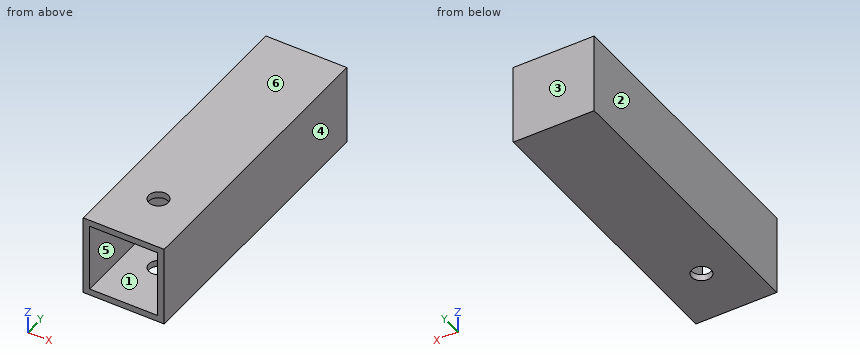
from build123d import *

# Parameters (mm, degrees)
SKETCH1_W                = 25.000000038
SKETCH1_H                = 25.000000038
BOSS_EXTRUDE1_DEPTH      = 120
SHELL1_T                 = -2
F_6_0_6_DIAMETER_HOLE1_D = 6
SKETCH6_W                = 35.234136461
SKETCH6_H                = 40.928418781
CUT_EXTRUDE1_DEPTH       = 48.26
SKETCH6_2_W              = 35.234136461
SKETCH6_2_H              = 40.928418781
CUT_EXTRUDE2_DEPTH       = 48.26
CUT_EXTRUDE2_DEPTH_BACK  = 48.26


with BuildPart() as part:
    # Sketch1 → Boss-Extrude1 (new body)
    with BuildSketch(Plane(origin=(0, 0, 0), x_dir=(1, 0, 0), z_dir=(0, 1, 0))):
        Rectangle(SKETCH1_W, SKETCH1_H)
    extrude(amount=BOSS_EXTRUDE1_DEPTH)

    # Shell1
    shell1_openings = [part.faces().sort_by_distance(p)[0] for p in [
        (0, 0, 0),
    ]]
    offset(amount=SHELL1_T, openings=shell1_openings, kind=Kind.INTERSECTION)

    # 6.0 _6_ Diameter Hole1 (through all)
    with Locations(Plane.XY.offset(12.500000019)):
        with Locations((0, 46.99999998)):
            Hole(F_6_0_6_DIAMETER_HOLE1_D / 2)

    # Sketch6 → Cut-Extrude1 (cut)
    with BuildSketch(Plane.XY):
        with Locations((1.431161847, 9.333336088)):
            Rectangle(SKETCH6_W, SKETCH6_H)
    extrude(amount=-CUT_EXTRUDE1_DEPTH, mode=Mode.SUBTRACT)

    # Sketch6_2 → Cut-Extrude2 (cut, two sides)
    with BuildSketch(Plane.XY) as cut_extrude2_sk:
        with Locations((1.431161847, 9.333336088)):
            Rectangle(SKETCH6_2_W, SKETCH6_2_H)
    extrude(amount=CUT_EXTRUDE2_DEPTH, mode=Mode.SUBTRACT)
    extrude(cut_extrude2_sk.sketch, amount=-CUT_EXTRUDE2_DEPTH_BACK, mode=Mode.SUBTRACT)


solid = part.part
Work out the finished part from the listing and answer in its coordinate system (mm). Face numbers are marked on the shaded views. A direction names the side the tool comes from. Round coordinates to 2 decimals unless told otherwise and drop trailing zeros. Write each loop counter-clockwise with the first axis right and the second up, starting at its lowest first coordinate (ties: lowest second). Pieces come first, ordered by that corner, then holes. Notation, with made-up numbers: M 85,49 L 126,49 A33 cw 126,85 Z; hole C -4.75,59 d5. An arc over 180 degrees is marked long. Use a Markdown table: item, result.
1) The part is cut by section A-A on x = 0. Give the vertices of the cut face in (y, z), plus the area to 3 significant figures.
Taken from the geometry:
| item | result |
|---|---|
| outline | M 29.8,-12.5 L 44,-12.5 L 44,-10.5 L 29.8,-10.5 Z; M 29.8,10.5 L 44,10.5 L 44,12.5 L 29.8,12.5 Z; M 50,-12.5 L 120,-12.5 L 120,12.5 L 50,12.5 L 50,10.5 L 118,10.5 L 118,-10.5 L 50,-10.5 Z |
| area | 379 mm2 |
2) Consider line 1 (Z direction, x = -10, y = 95.5); line 2 (Y direction, x = 0, z = -11.25); line 3 (X direction, y = 47, z = 11.45). Determine where each line is inside the solid, lowest interval first. Write a range as [from, to].
Taken from the geometry:
| item | result |
|---|---|
| line 1 | z = [-12.5, -10.5], [10.5, 12.5] |
| line 2 | y = [29.8, 44], [50, 120] |
| line 3 | x = [-12.5, -3], [3, 12.5] |
3) Which of the six approach directions +Z, -Z, +X, -X, +Y, -Y give full straight-line access (tool end or side, diameter ignored) to the marked faces 5 and 6?
Taken from the geometry:
| item | result |
|---|---|
| face 5 | -Y |
| face 6 | +Z, +X, -X, +Y, -Y |
4) The part is cut by section B-B on z = 4. Give the vertices of the cut face in (x, y).
Taken from the geometry:
| item | result |
|---|---|
| outline | M -12.5,29.8 L -10.5,29.8 L -10.5,118 L 10.5,118 L 10.5,29.8 L 12.5,29.8 L 12.5,120 L -12.5,120 Z |
5) The part is cut by section D-D on y = 47. Give the vertices of the cut face in (x, z), plus the area to 3 significant figures.
Taken from the geometry:
| item | result |
|---|---|
| outline | M -12.5,-12.5 L -3,-12.5 L -3,-10.5 L -10.5,-10.5 L -10.5,10.5 L -3,10.5 L -3,12.5 L -12.5,12.5 Z; M 3,-12.5 L 12.5,-12.5 L 12.5,12.5 L 3,12.5 L 3,10.5 L 10.5,10.5 L 10.5,-10.5 L 3,-10.5 Z |
| area | 160 mm2 |
6) Determine the mould class of the marked faces 1, 2, 3 and 4 for opening direction X: pulls with the +X half, pulls with the -X half, needs draft (parallel to the pull), parting line crosses it, or undercut.
Taken from the geometry:
| item | result |
|---|---|
| face 1 | undercut |
| face 2 | pulls with the -X half |
| face 3 | needs draft |
| face 4 | pulls with the +X half |
7) Flat-ended cylindrical pins translate along their axes: pin 1 (1.5 mm diameter, centred on x = 0.5, z = 6.5, fed in from -Y); pin 2 (7 mm diameter, centred on x = 0, y = 47, fed in from -Z). Find the tip coordinate at first contact, or state that the pin passes through.
Taken from the geometry:
| item | result |
|---|---|
| pin 1 | stops at y = 118 |
| pin 2 | stops at z = -12.5 |
8) The part is cut by section C-C on y = 58. Give the vertices of the cut face in (x, z), plus the area to 3 significant figures.
Taken from the geometry:
| item | result |
|---|---|
| outline | M -12.5,-12.5 L 12.5,-12.5 L 12.5,12.5 L -12.5,12.5 Z; hole M -10.5,-10.5 L 10.5,-10.5 L 10.5,10.5 L -10.5,10.5 Z |
| area | 184 mm2 |
